Autodesk Inventor part; units mm, degrees
ref_plane "YZ Plane" through (0, 0, 0) normal (1, 0, 0) x (0, 1, 0)
ref_plane "XZ Plane" through (0, 0, 0) normal (0, 1, 0) x (-1, 0, 0)
ref_plane "XY Plane" through (0, 0, 0) normal (0, 0, 1) x (1, 0, 0)
sketch "スケッチ1" plane through (0, 0, 0) normal (0, 1, 0) x (-1, 0, 0)
  line L0 (11, 11) -> (-11, 11)
  line L1 (-11, 11) -> (-11, -9.8801)
  line L2 (11, -9) -> (11, 11)
  line L3 (-11, -5.4423) -> (-11, -109)
  line L4 (-11, -109) -> (11, -109)
  line L5 (11, -109) -> (11, -9)
  circle A0 centre (0, 0) radius 11
  point P0 (11, 1)
  dimension "d1" = 20
  dimension "d12" = 22
  dimension "d13" = 120
extrude "押し出し1" add sketch "スケッチ1" along normal blind 2.5
sketch "スケッチ2" plane through (0, 0, 0) normal (0, -1, 0) x (1, 0, 0)
  line L0 (11, 11) -> (-11, 11)
  line L1 (-11, 11) -> (-11, -14)
  line L2 (-11, -14) -> (11, -14)
  line L3 (11, -14) -> (11, 11)
  line L4 (4, -14) -> (-4, -14)
  line L5 (-4, -14) -> (-4, -9)
  line L6 (-4, -9) -> (4, -9)
  line L7 (4, -9) -> (4, -14)
  point P0 (0, 0)
  point P1 (0, -14)
  dimension "d14" = 25
  dimension "d15" = 8
  dimension "d16" = 5
extrude "押し出し2" cut sketch "スケッチ2" against normal through all contours L3 L2 L7 L6 L5 L1 L0
sketch "スケッチ3" plane through (0, 2.5, 0) normal (0, 1, 0) x (1, 0, 0)
  line L0 (4, 19) -> (6.5, 19)
  line L1 (6.5, 19) -> (6.5, 29)
  line L2 (6.5, 29) -> (4, 29)
  line L3 (4, 29) -> (4, 19)
  line L4 (4, 14) -> (11, 14)
  line L5 (4, 9) -> (4, 14)
  point P0 (0, 0)
  dimension "d19" = 2.5
  dimension "d20" = 10
  dimension "d21" = 5
extrude "押し出し3" cut sketch "スケッチ3" against normal through all
equation "\"BendRadius\" = Thickness"
equation "\"BendReliefWidth\" = Thickness"
equation "\"BendReliefDepth\" = 0.5 * Thickness"
equation "\"CornerReliefSize\" = 4 * Thickness"
equation "\"MinimumRemnant\" = 2 * Thickness"
equation "\"TransitionRadius\" = BendRadius"
equation "\"JacobiRadiusSize\" = BendRadius"
equation "\"GapSize\" = Thickness"
properties part number "dish_upper" material "木材 (カエデ材)"
For this review, take the finished solid that the model builds, in its own axes (mm). A direction names the side the tool comes from. Round coordinates to 2 decimals unless told otherwise and drop trailing zeros. Write each loop counter-clockwise with the first axis right and the second up, starting at its lowest first coordinate (ties: lowest second). Pieces come first, ordered by that corner, then holes. Notation, with made-up numbers: (83, 47.5) -> (87, 47.5) arc R15 cw to (87, 56.5) -> close; hole circle Ø1 at (38, 1.5). An arc over 180 degrees is marked (long way). One line per question, with ' | ' between items. Start each with the question number.
(1) Add section A-A, the plane y = 1.8. Write out the cut boundary in (x, z).
(2) Mouldability with a two-part tool opening along X and no side actions: class faces 5 (the face through (-4, 1, -12)), 6 (the face through (5, 1, -29)), 7 (the face through (0, 1, -9)) as released by +X, released by -X, zero draft, split by the parting line, or undercut.
(3) Add section B-B, the plane z = -27.5. Write out the cut boundary in (x, y).
(4) For line 1 along Z through (x, y) = (-4.5, 0.35); line 2 along Z through (x, y) = (4.25, 1.05), list the stretches that pass through material, from the lowest coordinate up. Write a range as from..to.
(5) Insertion check: P1, Ø1.2, axis at y = 0.5, z = -11, coming from the +X side; P2, Ø0.8, axis at x = 5.5, y = 1.5, coming from the +Z side; P3, Ø4, axis at x = 5.5, z = -68.5, coming from the -Y side. Each pin has a flat end and moves straight along its axis. Give the tip position at first contact, or say it passes through.
(6) Add section C-C, the plane x = -8.5. Write out the cut boundary in (y, z), plus the area to 4 significant figures.
(7) Tool access review of faces 1 (the face through (-11, 1, -62)), 2 (the face through (6.5, 1, -24)), 3 (the face through (-8, 1, -14)), 4 (the face through (7, 1, -14)): name each direction out of +Z, -Z, +X, -X, +Y, -Y from which nothing blocks a thin tool from reaching the whole face with its end or side.
Answer list:
1) outline: (-11, -109) -> (11, -109) -> (11, -14) -> (4, -14) -> (4, -9) -> (-4, -9) -> (-4, -14) -> (-11, -14) -> close; hole (4, -29) -> (6.5, -29) -> (6.5, -19) -> (4, -19) -> close
2) face 5: released by -X | face 6: undercut | face 7: zero draft
3) outline: (-11, 0) -> (4, 0) -> (4, 2.5) -> (-11, 2.5) -> close; (6.5, 0) -> (11, 0) -> (11, 2.5) -> (6.5, 2.5) -> close
4) line 1: -109..-14 | line 2: -109..-29, -19..-14
5) P1: x = 4 | P2: z = -14 | P3: y = 0
6) outline: (0, -109) -> (2.5, -109) -> (2.5, -14) -> (0, -14) -> close | area: 237.5 mm²
7) face 1: +Z, -Z, -X, +Y, -Y | face 2: +Y, -Y | face 3: +Z, -X, +Y, -Y | face 4: +Z, +X, +Y, -Y
